from build123d import *

# Parameters (mm, degrees)
SKETCH083_R   = 5
SKETCH083_R_2 = 2.75
PAD063_DEPTH  = 4.5
PAD064_DEPTH  = 9
SKETCH085_W   = 0.5
SKETCH085_H   = 3
PAD065_DEPTH  = 4


with BuildPart() as part:
    # Sketch083 → Pad063 (new body)
    with BuildSketch(Plane.XY):
        Circle(SKETCH083_R)
        Circle(SKETCH083_R_2, mode=Mode.SUBTRACT)
    extrude(amount=PAD063_DEPTH)

    # Sketch084 → Pad064 (join)
    with BuildSketch(Plane.XY):
        with BuildLine():
            ThreePointArc((3.3, 1.781151), (0, 3.75), (-3.3, 1.781151))
            Line((-3.3, -1.781151), (-3.3, 1.781151))
            ThreePointArc((-3.3, -1.781151), (0, -3.75), (3.3, -1.781151))
            Line((3.3, 1.781151), (3.3, -1.781151))
        make_face()
    extrude(amount=-PAD064_DEPTH)

    # Sketch085 → Pad065 (join)
    with BuildSketch(Plane.XY.offset(-9)):
        with Locations((-2.5, 0)):
            Rectangle(SKETCH085_W, SKETCH085_H)
        with Locations((2.5, 0)):
            Rectangle(SKETCH085_W, SKETCH085_H)
    extrude(amount=-PAD065_DEPTH)


solid = part.part
Input: part model. Units: mm. Frame: model coordinates. A direction names the side the tool comes from. Give positions to 0.01 mm unless a question says otherwise; leave off trailing zeros. Write each loop counter-clockwise with the first axis right and the second up, starting at its lowest first coordinate (ties: lowest second). Pieces come first, ordered by that corner, then holes. Notation, with made-up numbers: M 83.5,57.5 L 128.5,57.5 A30 ccw 128.5,83.5 Z; hole C 7,-5.75 d6. An arc over 180 degrees is marked long. Use one line per item in the form item = value.
1. Mould query, pull axis Y, two halves, no side actions, for faces 4 (the face through (0, 0, 0)), 5 (the face through (-1.08, -4.88, 2.22)), 6 (the face through (-2.75, 0, -11)). Classes: released by +Y, released by -Y, zero draft, split by the parting line, or undercut.
Outcome:
face_4 = undercut
face_5 = split by the parting line
face_6 = zero draft
2. First-contact query: P1, Ø2, axis at x = 2.5, z = 2.5, coming from the +Y side; P2, Ø1.8, axis at y = 0.5, z = -5, coming from the +X side; P3, Ø0.9, axis at y = 0, z = -10, coming from the -X side. Flat tips, straight axial feed; report the tip coordinate or a pass-through.
Outcome:
P1 = 4.77
P2 = 3.3
P3 = -2.75
3. Ray query, L1, parallel to Y at x = 0, z = 2; L2, parallel to Z at x = -1.75, y = 1; L3, parallel to Z at x = -3.5, y = 2.5. Return the intervals inside material, ascending.
Outcome:
L1 = -5 to -2.75, 2.75 to 5
L2 = -9 to 0
L3 = 0 to 4.5
4. Reachability of faces 1 (the face through (-2.3, -3.3, 0)), 2 (the face through (0.06, 3.75, -4.44)), 3 (the face through (3.3, 0, -4)) from +Z, -Z, +X, -X, +Y, -Y: full face, straight path, thin tool, end or side. Return the list, or none.
Outcome:
face_1 = -Z
face_2 = -Z, +Y
face_3 = -Z, +X, +Y, -Y
5. Cut plane B-B on x = -3. Return loops of the section in (y, z), and give its area (3 significant figures).
Outcome:
outline = M -4,0 L -2.25,0 L -2.25,-9 L 2.25,-9 L 2.25,0 L 4,0 L 4,4.5 L -4,4.5 Z
area = 76.5 mm²
6. Cut plane A-A on z = -11.5. Return loops of the section in (x, y).
Outcome:
outline = M -2.75,-1.5 L -2.25,-1.5 L -2.25,1.5 L -2.75,1.5 Z; M 2.25,-1.5 L 2.75,-1.5 L 2.75,1.5 L 2.25,1.5 Z
7. Cut plane D-D on x = 0. Return loops of the section in (y, z), and give its area (4 significant figures).
Outcome:
outline = M -5,0 L -3.75,0 L -3.75,-9 L 3.75,-9 L 3.75,0 L 5,0 L 5,4.5 L 2.75,4.5 L 2.75,0 L -2.75,0 L -2.75,4.5 L -5,4.5 Z
area = 87.75 mm²
8. Cut plane C-C on y = 0. Return loops of the section in (x, z).
Outcome:
outline = M -5,0 L -3.3,0 L -3.3,-9 L -2.75,-9 L -2.75,-13 L -2.25,-13 L -2.25,-9 L 2.25,-9 L 2.25,-13 L 2.75,-13 L 2.75,-9 L 3.3,-9 L 3.3,0 L 5,0 L 5,4.5 L 2.75,4.5 L 2.75,0 L -2.75,0 L -2.75,4.5 L -5,4.5 Z
